Check sheet for the modelled part. Datum: model origin and axes. Units: mm. A direction names the side the tool comes from. Give positions to 0.01 mm unless a question says otherwise; leave off trailing zeros. Write each loop counter-clockwise with the first axis right and the second up, starting at its lowest first coordinate (ties: lowest second). Pieces come first, ordered by that corner, then holes.
from build123d import *

# Parameters (mm, degrees)
SKETCH1_R           = 70
BOSS_EXTRUDE1_DEPTH = 40
SKETCH2_R           = 7.5
CUT_EXTRUDE1_DEPTH  = 30
CIRPATTERN1_COUNT   = 4


with BuildPart() as part:
    # Sketch1 → Boss-Extrude1 (new body)
    with BuildSketch(Plane(origin=(0, 0, 0), x_dir=(1, 0, 0), z_dir=(0, 1, 0))):
        with BuildLine():
            Line((95.123177318, 30.847708779), (185, 15))
            Line((185, 15), (235, 15))
            Line((235, 15), (235, -15))
            Line((235, -15), (185, -15))
            Line((185, -15), (95.123177318, -30.847708779))
            ThreePointArc((95.123177318, -30.847708779), (70.710678119, -70.710678119), (30.847708779, -95.123177318))
            Line((30.847708779, -95.123177318), (15, -185))
            Line((15, -185), (15, -235))
            Line((15, -235), (-15, -235))
            Line((-15, -235), (-15, -185))
            Line((-15, -185), (-30.847708779, -95.123177318))
            ThreePointArc((-30.847708779, -95.123177318), (-70.710678119, -70.710678119), (-95.123177318, -30.847708779))
            Line((-95.123177318, -30.847708779), (-185, -15))
            Line((-185, -15), (-235, -15))
            Line((-235, -15), (-235, 15))
            Line((-235, 15), (-185, 15))
            Line((-185, 15), (-95.123177318, 30.847708779))
            ThreePointArc((-95.123177318, 30.847708779), (-70.710678119, 70.710678119), (-30.847708779, 95.123177318))
            Line((-30.847708779, 95.123177318), (-15, 185))
            Line((-15, 185), (-15, 235))
            Line((-15, 235), (15, 235))
            Line((15, 235), (15, 185))
            Line((15, 185), (30.847708779, 95.123177318))
            ThreePointArc((30.847708779, 95.123177318), (70.710678119, 70.710678119), (95.123177318, 30.847708779))
        make_face()
        Circle(SKETCH1_R, mode=Mode.SUBTRACT)
    extrude(amount=BOSS_EXTRUDE1_DEPTH)

    # Sketch2 → Cut-Extrude1 (cut)
    with BuildSketch(Plane.XY.offset(235)):
        with Locations((0, 20)):
            Circle(SKETCH2_R)
    cut_extrude1 = extrude(amount=-CUT_EXTRUDE1_DEPTH, mode=Mode.SUBTRACT)

    # CirPattern1: Cut-Extrude1 ×4 about axis
    cirpattern1_axis = Axis((0, 0, 0), (0, 1, 0))
    for i in range(1, CIRPATTERN1_COUNT):
        add(cut_extrude1.rotate(cirpattern1_axis, i * 360 / CIRPATTERN1_COUNT), mode=Mode.SUBTRACT)


solid = part.part
1) Sectioned sample at A-A on x = 0. Record the boundary of the cut face in (y, z).
2) Draft check along Z on faces 5 (the flat face through (0, 20, -205)), 6 (the flat face through (7, 15, 235)), 7 (the cylindrical face through (220.21, 27.436, 0.976)), 8 (the flat face through (205, 20, 0)). Enter one of: +Z half, -Z half, draft (parallel to the pull), parting line (faces both ways), or undercut.
3) Sectioned sample at C-C on y = 6.5. Record the boundary of the cut face in (x, z), then the cut area to 3 significant figures.
4) Sectioned sample at B-B on z = 0. Record the boundary of the cut face in (x, y), then the cut area to 3 significant figures.
5) Sectioned sample at D-D on z = 54. Record the boundary of the cut face in (x, y).
6) Scan lines: L1, parallel to Z at x = 3, y = 36.5; L2, parallel to Y at x = 0, z = -224; L3, parallel to Z at x = 1.5, y = 27.5. Record each from-to range of solid material in increasing order.
7) Access from +Z, -Z, +X, -X, +Y, -Y to the whole of each face (thin tool, end or side, straight path). Record for faces 1 (the flat face through (15, 20, -210)), 2 (the flat face through (-210, 20, 15)), 3 (the flat face through (-210, 20, -15)), 4 (the flat face through (210, 20, 15)).
8) Gauge pin test, flat ends, axial feed: pin 1 (12 mm diameter, centred on x = -203, y = 28, fed in from -Z); pin 2 (20 mm diameter, centred on y = 28.5, z = -206.5, fed in from -X); pin 3 (4.5 mm diameter, centred on y = 23, z = -0.5, fed in from -X). Record the tip position at first contact, or that the pin passes through.
Answers below:
1. outline: (0, -235) - (12.5, -235) - (12.5, -205) - (27.5, -205) - (27.5, -235) - (40, -235) - (40, -70) - (0, -70) - close; (0, 70) - (40, 70) - (40, 235) - (27.5, 235) - (27.5, 205) - (12.5, 205) - (12.5, 235) - (0, 235) - close
2. face 5: -Z half
2. face 6: +Z half
2. face 7: undercut
2. face 8: undercut
3. outline: (-235, -15) - (-185, -15) - (-95.12, -30.85) arc R100 ccw to (-30.85, -95.12) - (-15, -185) - (-15, -235) - (15, -235) - (15, -185) - (30.85, -95.12) arc R100 ccw to (95.12, -30.85) - (185, -15) - (235, -15) - (235, 15) - (185, 15) - (95.12, 30.85) arc R100 ccw to (30.85, 95.12) - (15, 185) - (15, 235) - (-15, 235) - (-15, 185) - (-30.85, 95.12) arc R100 ccw to (-95.12, 30.85) - (-185, 15) - (-235, 15) - close; hole circle Ø140 at (0, 0)
3. area: 37,700 mm2
4. outline: (-235, 0) - (-70, 0) - (-70, 40) - (-235, 40) - (-235, 27.5) - (-205, 27.5) - (-205, 12.5) - (-235, 12.5) - close; (70, 0) - (235, 0) - (235, 12.5) - (205, 12.5) - (205, 27.5) - (235, 27.5) - (235, 40) - (70, 40) - close
4. area: 12,300 mm2
5. outline: (-84.17, 0) - (-44.54, 0) - (-44.54, 40) - (-84.17, 40) - close; (44.54, 0) - (84.17, 0) - (84.17, 40) - (44.54, 40) - close
6. L1: z = -235 to -69.94, 69.94 to 235
6. L2: y = 0 to 12.5, 27.5 to 40
6. L3: z = -235 to -69.98, 69.98 to 235
7. face 1: -Z, +X, +Y, -Y
7. face 2: +Z, -X, +Y, -Y
7. face 3: -Z, -X, +Y, -Y
7. face 4: +Z, +X, +Y, -Y
8. pin 1: stops at z = -15
8. pin 2: stops at x = -15
8. pin 3: stops at x = -205
